```python
from build123d import *
from build123d.topology import SkipClean

# Parameters (mm, degrees)
SKETCH1_W                = 26
SKETCH1_H                = 10
SKETCH1_R                = 1.5
SKETCH1_R_2              = 1
MAINBODY_DEPTH           = 4
PUSHEXTRUSION_DEPTH      = 5
PUSHEXTRUSION_DEPTH_BACK = 1
PUSHEXTRUSION_START      = 4
SKETCH1_5_R              = 2.5
SKETCH1_6_W              = 20
SKETCH1_6_H              = 4
SKETCH1_6_R              = 1.5
SKETCH1_6_R_2            = 1
CUT_EXTRUDE1_DEPTH       = 2.5
BOSS_EXTRUDE1_START      = 4
SKETCH1_7_W              = 19
SKETCH1_7_H              = 10
SKETCH1_7_R              = 2.5
BOSS_EXTRUDE1_DEPTH      = 1


with BuildPart() as part:
    # Sketch1 → MainBody (new body)
    with BuildSketch(Plane(origin=(0, 0, 0), x_dir=(1, 0, 0), z_dir=(0, 1, 0))):
        with Locations((13, 5)):
            Rectangle(SKETCH1_W, SKETCH1_H)
        with Locations(Location((6.5, 5, 0), (0, 0, 270))):
            Circle(SKETCH1_R, mode=Mode.SUBTRACT)
        with BuildLine():
            ThreePointArc((5, 9), (5.398014876, 8.980148761), (5.792079208, 8.920792079))
            Line((5.792079208, 8.920792079), (5, 9))
        make_face(mode=Mode.SUBTRACT)
        with BuildLine():
            ThreePointArc((5.792079208, 1.079207921), (5.398014876, 1.019851239), (5, 1))
            Line((5, 1), (5.792079208, 1.079207921))
        make_face(mode=Mode.SUBTRACT)
        with Locations(Location((16.5, 5, 0), (0, 0, 270))):
            Circle(SKETCH1_R_2, mode=Mode.SUBTRACT)
        with Locations(Location((22.5, 5, 0), (0, 0, 270))):
            Circle(SKETCH1_R_2, mode=Mode.SUBTRACT)
    extrude(amount=MAINBODY_DEPTH)

    # Sketch1<6> → Cut-Extrude1 (cut)
    # profile 1 of 4: a face of its own
    with SkipClean():  # the faces are left unmerged after this step: merging them gives an invalid solid
        with BuildSketch(Plane(origin=(0, 0, 0), x_dir=(1, 0, 0), z_dir=(0, 1, 0))):
            with Locations((15, 5)):
                Rectangle(SKETCH1_6_W, SKETCH1_6_H)
            with Locations(Location((6.5, 5, 0), (0, 0, 270))):
                Circle(SKETCH1_6_R, mode=Mode.SUBTRACT)
            with Locations(Location((16.5, 5, 0), (0, 0, 270))):
                Circle(SKETCH1_6_R_2, mode=Mode.SUBTRACT)
            with Locations(Location((22.5, 5, 0), (0, 0, 270))):
                Circle(SKETCH1_6_R_2, mode=Mode.SUBTRACT)
        # profile 2 of 4: a face of its own
        with BuildSketch(Plane(origin=(0, 0, 0), x_dir=(1, 0, 0), z_dir=(0, 1, 0))):
            Polygon((25, 7), (5, 9), (5, 7), align=None)
        # profile 3 of 4: a face of its own
        with BuildSketch(Plane(origin=(0, 0, 0), x_dir=(1, 0, 0), z_dir=(0, 1, 0))):
            Polygon((25, 3), (5, 1), (5, 3), align=None)
        # profile 4 of 4: a face of its own
        with BuildSketch(Plane(origin=(0, 0, 0), x_dir=(1, 0, 0), z_dir=(0, 1, 0))):
            with BuildLine():
                Line((5, 5), (5, 7))
                Line((5, 7), (5, 9))
                ThreePointArc((5, 9), (1, 5), (5, 1))
                Line((5, 1), (5, 3))
                Line((5, 3), (5, 5))
            make_face()
        extrude(amount=CUT_EXTRUDE1_DEPTH, mode=Mode.SUBTRACT)



with BuildPart() as body_2:
    # Sketch1<5> → PushExtrusion (new, two sides: drawn at the far end of the back side and taken through both)
    with BuildSketch(Plane(origin=(0, 0, 0), x_dir=(1, 0, 0), z_dir=(0, 1, 0)).offset(PUSHEXTRUSION_START - PUSHEXTRUSION_DEPTH_BACK)):
        with Locations(Location((42, 5, 0), (0, 0, 270))):
            Circle(SKETCH1_5_R)
    extrude(amount=PUSHEXTRUSION_DEPTH + PUSHEXTRUSION_DEPTH_BACK)


with BuildPart() as part_1:
    with SkipClean():  # the faces are left unmerged after this step: merging them gives an invalid solid
        add(part.part)

        add(body_2.part)  # Boss-Extrude1 merges body 2
        # Sketch1<7> → Boss-Extrude1 (add)
        with BuildSketch(Plane(origin=(0, 0, 0), x_dir=(1, 0, 0), z_dir=(0, 1, 0)).offset(BOSS_EXTRUDE1_START)):
            with Locations((35.5, 5)):
                Rectangle(SKETCH1_7_W, SKETCH1_7_H)
            with Locations(Location((42, 5, 0), (0, 0, 270))):
                Circle(SKETCH1_7_R, mode=Mode.SUBTRACT)
        extrude(amount=-BOSS_EXTRUDE1_DEPTH)


solid = part_1.part
```
Check sheet for the modelled part. Datum: model origin and axes. Units: mm. A direction names the side the tool comes from. Round coordinates to 2 decimals unless told otherwise and drop trailing zeros. Write each loop counter-clockwise with the first axis right and the second up, starting at its lowest first coordinate (ties: lowest second). Pieces come first, ordered by that corner, then holes. Notation, with made-up numbers: M 61.5,-8.5 L 119.5,-8.5 A20 cw 119.5,0.5 Z; hole C 18,-17 d2. An arc over 180 degrees is marked long. Write item = value, one per line. Start each with the question number.
1. Section check B-B, the plane x = 13.5. Record the cut outline in (y, z), then the cut area to 4 significant figures.
2. Section check C-C, the plane z = -5.5. Record the cut outline in (x, y).
3. Tool access check on faces 5 (the flat face through (42, 9, -5)), 6 (the flat face through (35, 3, -5)), 7 (the flat face through (13, 2.5, -5)). Record the directions out of +Z, -Z, +X, -X, +Y, -Y that give a thin tool (end or side, any length) a straight path to the whole face; none if there is none.
4. Section check D-D, the plane y = 5. Record the cut outline in (x, z).
5. Section check A-A, the plane x = 22.5. Record the cut outline in (y, z).
6. Scan lines: line 1 (X direction, y = 2.9, z = -5); line 2 (X direction, y = 3.45, z = -5); line 3 (Z direction, x = 6.5, y = 2.9). Record each from-to range of solid material in increasing order. Write a range as [from, to].
7. Gauge pin test, flat ends, axial feed: pin 1 (1.5 mm diameter, centred on x = 36.5, z = -3.5, fed in from +Y); pin 2 (0.9 mm diameter, centred on y = 1, z = -3, fed in from +X); pin 3 (3 mm diameter, centred on x = 22.5, z = -5, fed in from -Y). Record the tip position at first contact, or that the pin passes through.
8. Release check for a two-part mould opening along X. For faces 1 (the flat face through (22.2, 4, -6.2)), 2 (the flat face through (45, 3.5, -4.9)), 3 (the cylindrical face through (39.56, 6.46, -5.54)), 4 (the flat face through (15.53, 1.232, -7.947)) record: pulls with the +X half, pulls with the -X half, needs draft (parallel to the pull), parting line crosses it, or undercut.
Results found:
q1.outline = M 0,-10 L 4,-10 L 4,0 L 0,0 L 0,-1.85 L 2.5,-1.85 L 2.5,-8.15 L 0,-8.15 Z
q1.area = 24.25 mm^2
q2.outline = M 0,0 L 1.03,0 L 1.03,2.5 L 5.09,2.5 L 5.09,4 L 0,4 Z; M 7.91,2.5 L 15.63,2.5 L 15.63,4 L 7.91,4 Z; M 17.37,2.5 L 21.63,2.5 L 21.63,4 L 17.37,4 Z; M 23.37,2.5 L 25,2.5 L 25,0 L 26,0 L 26,3 L 45,3 L 45,4 L 44.45,4 L 44.45,9 L 39.55,9 L 39.55,4 L 23.37,4 Z
q3.face_5 = +Z, -Z, +X, -X, +Y
q3.face_6 = +Z, -Z, +X, -Y
q3.face_7 = -Y
q4.outline = C 42,-5 d5
q5.outline = M 0,-10 L 4,-10 L 4,-6 L 2.5,-6 L 2.5,-7.25 L 0,-7.25 Z; M 0,-2.75 L 2.5,-2.75 L 2.5,-4 L 4,-4 L 4,0 L 0,0 Z
q6.line_1 = [0, 5], [8, 15.5], [17.5, 21.5], [23.5, 26]
q6.line_2 = [0, 5], [8, 15.5], [17.5, 21.5], [23.5, 45]
q6.line_3 = [-10, -6.5], [-3.5, 0]
q7.pin_1 = 4
q7.pin_2 = 26
q7.pin_3 = 2.5
q8.face_1 = needs draft
q8.face_2 = pulls with the +X half
q8.face_3 = parting line crosses it
q8.face_4 = undercut
